The listing builds one solid part. Answer for the finished solid, in the listing's coordinates (mm). Coordinates: 2 decimals unless noted, no trailing zeros. Order: outer loops, then holes, each group sorted by start corner. A loop starts at its lowest first (then second) coordinate and runs counter-clockwise, first axis right, second up.
```python
from build123d import *

# Parameters (mm, degrees)
SKETCH011_W     = 6
SKETCH011_H     = 6
SKETCH011_R     = 1.6
PAD003_DEPTH    = 1
POCKET007_DEPTH = 6.001
POCKET008_DEPTH = 6
FILLET002_R     = 0.25
FILLET003_R     = 0.1


with BuildPart() as part:
    # Sketch011 → Pad003 (new body)
    with BuildSketch(Plane.XY.offset(8.5)):
        with Locations((-4.125, 0)):
            Rectangle(SKETCH011_W, SKETCH011_H)
        with Locations((-4.125, 0)):
            Circle(SKETCH011_R, mode=Mode.SUBTRACT)
    extrude(amount=PAD003_DEPTH)

    # Sketch012 → Pocket007 (cut, through all)
    with BuildSketch(Plane(origin=(0, -3, 8.5), x_dir=(1, 0, 0), z_dir=(0, -1, 0))):
        with BuildLine():
            ThreePointArc((-1.125, 0.5), (-4.125, 1), (-7.125, 0.5))
            Line((-7.740595, 0.5), (-7.125, 0.5))
            Line((-7.740595, 1.84364), (-7.740595, 0.5))
            Line((-7.740595, 1.84364), (-0.509405, 1.84364))
            Line((-0.509405, 1.84364), (-0.509405, 0.5))
            Line((-0.509405, 0.5), (-1.125, 0.5))
        make_face()
    extrude(amount=-POCKET007_DEPTH, mode=Mode.SUBTRACT)

    # Sketch013 → Pocket008 (cut)
    with BuildSketch(Plane(origin=(-7.125, 0, 8.5), x_dir=(0, -1, 0), z_dir=(-1, 0, 0))):
        with BuildLine():
            ThreePointArc((3, 0.5), (0, 1), (-3, 0.5))
            Line((-3.32758, 0.5), (-3, 0.5))
            Line((-3.32758, 1.60662), (-3.32758, 0.5))
            Line((-3.32758, 1.60662), (3.32758, 1.60662))
            Line((3.32758, 1.60662), (3.32758, 0.5))
            Line((3.32758, 0.5), (3, 0.5))
        make_face()
    extrude(amount=-POCKET008_DEPTH, mode=Mode.SUBTRACT)

    # Fillet002
    fillet002_edges = [part.edges().sort_by_distance(p)[0] for p in [
        (-7.125, -3, 8.75),
        (-7.125, 3, 8.75),
        (-1.125, -3, 8.75),
        (-1.125, 3, 8.75),
    ]]
    fillet(fillet002_edges, radius=FILLET002_R)

    # Fillet003
    fillet003_edges = [part.edges().sort_by_distance(p)[0] for p in [
        (-7.125, 0, 8.5),
    ]]
    fillet(fillet003_edges, radius=FILLET003_R)


solid = part.part
```
1) A cutting plane is placed at A-A, the plane z = 8.8. Write down the section's boundary in (x, y) (3 decimals), plus the area to 3 significant figures.
2) A cutting plane is placed at C-C, the plane y = 1. Write down the section's boundary in (x, z) (3 decimals).
3) The mould has two halves that part along Y. Classify faces 1 (the cylindrical face through (-2.647, -0.613, 8.959)), 2 (the flat face through (-5.5, -1.2, 8.5)), 3 (the cylindrical face through (-4.17, -2.3, 9.21)), 4 (the cylindrical face through (-4.166, 2.271, 9.217)): released by +Y, released by -Y, zero draft, split by the parting line, or undercut.
4) Each of these flat-tipped pins is pushed along its axis until it touches: P1, Ø1.5, axis at x = -3.5, y = 1, coming from the +Z side; P2, Ø3, axis at x = -4.125, y = 0, coming from the +Z side. Where does it stop, or does it pass through?
5) A cutting plane is placed at B-B, the plane x = -3.75. Write down the section's boundary in (y, z), plus the area to 3 significant figures.
6) Straight lines are drawn through the part: probe 1 along X at (y, z) = (0, 8.9) (3 decimals); probe 2 along Z at (x, y) = (-2.25, 0); probe 3 along X at (y, z) = (-1, 8.8) (3 decimals). For each, find the intervals that lie inside material, in ascending order.
7) A cutting plane is placed at D-D, the plane y = -2.5. Write down the section's boundary in (x, z) (3 decimals), plus the area to 3 significant figures.
Working result:
1. outline: (-7.125, -2.75) arc R0.25 ccw to (-6.875, -3) - (-1.375, -3) arc R0.25 ccw to (-1.125, -2.75) - (-1.125, 2.75) arc R0.25 ccw to (-1.375, 3) - (-6.875, 3) arc R0.25 ccw to (-7.125, 2.75) - close; hole circle Ø3.2 at (-4.125, 0)
1. area: 27.9 mm2
2. outline: (-7.125, 8.6) arc R0.1 ccw to (-7.025, 8.5) - (-5.374, 8.5) - (-5.374, 9.415) arc R9.25 ccw to (-7.125, 9) - close; (-2.876, 8.5) - (-1.225, 8.5) arc R0.1 ccw to (-1.125, 8.6) - (-1.125, 9) arc R9.25 ccw to (-2.876, 9.415) - close
3. face 1: undercut
3. face 2: zero draft
3. face 3: released by -Y
3. face 4: released by +Y
4. P1: stops at z = 9.43
4. P2: passes through
5. outline: (-3, 8.6) arc R0.1 ccw to (-2.9, 8.5) - (-1.56, 8.5) - (-1.56, 9.37) arc R9.25 ccw to (-3, 9) - close; (1.56, 8.5) - (2.9, 8.5) arc R0.1 ccw to (3, 8.6) - (3, 9) arc R9.25 ccw to (1.56, 9.37) - close
5. area: 2.03 mm2
6. probe 1: x = -7.125 to -5.725, -2.525 to -1.125
6. probe 2: z = 8.5 to 9.31
6. probe 3: x = -7.125 to -5.374, -2.876 to -1.125
7. outline: (-7.125, 8.6) arc R0.1 ccw to (-7.025, 8.5) - (-1.225, 8.5) arc R0.1 ccw to (-1.125, 8.6) - (-1.125, 9) arc R9.25 ccw to (-1.625, 9.156) - (-6.625, 9.156) arc R9.25 ccw to (-7.125, 9) - close
7. area: 3.85 mm2
